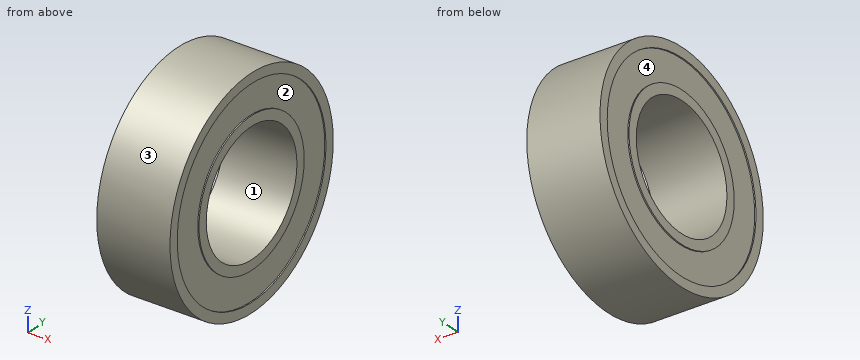
Autodesk Inventor part; units mm, degrees
ref_plane "YZ Plane" through (0, 0, 0) normal (1, 0, 0) x (0, 1, 0)
ref_plane "XZ Plane" through (0, 0, 0) normal (0, 1, 0) x (-1, 0, 0)
ref_plane "XY Plane" through (0, 0, 0) normal (0, 0, 1) x (1, 0, 0)
sketch "Эскиз1" plane through (0, 0, 0) normal (1, 0, 0) x (0, 1, 0)
  circle A0 centre (0, 0) radius 2.5
  circle A1 centre (0, 0) radius 4.5
  circle A2 centre (0, 0) radius 2.9
  circle A3 centre (0, 0) radius 4.1
  dimension "d0" = 5
  dimension "d1" = 9
  dimension "d2" = 0.4
  dimension "d3" = 0.4
extrude "Выдавливание1" add sketch "Эскиз1" along normal mid plane 3
extrude "Выдавливание2" add sketch "Эскиз1" along normal mid plane 2.9 contours A3
properties part number "roller_5_9_3"
Geometry check sheet. Reference: the model listing, model coordinates, mm. Face numbers are marked on the shaded views. A direction names the side the tool comes from. Round coordinates to 2 decimals unless told otherwise and drop trailing zeros. Order: outer loops, then holes, each group sorted by start corner. A loop starts at its lowest first (then second) coordinate and runs counter-clockwise, first axis right, second up. Notation, with made-up numbers: M 13,-7.75 L 53,-7.75 A27 cw 53,16.25 Z; hole C 72,76.5 d11. An arc over 180 degrees is marked long. Answer in a Markdown table with one row per item. Add a question column.
Item 1: Sectioned sample at C-C, the plane x = 0.75. Enter the section's corners in (y, z), plus the area to 3 significant figures.
Item 2: Set-up check for the marked faces 1 and 2: record each of +Z, -Z, +X, -X, +Y, -Y from which the full face is reachable in a straight line by a thin tool's end or side.
Item 3: Sectioned sample at D-D, the plane z = 3.75. Enter the section's corners in (x, y), plus the area to 3 significant figures.
Item 4: Sectioned sample at A-A, the plane y = 0. Enter the section's corners in (x, z), plus the area to 3 significant figures.
Item 5: Material ranges on L1, parallel to X at y = 2.25, z = 3; L2, parallel to Z at x = 1.3, y = -1.5; L3, parallel to Y at x = 0.1, z = -0.5, recorded low to high. Write a range as [from, to].
Item 6: Depth check by flat-ended pin: pin 1 Ø1.5 at (y, z) = (1, -0.5) entering from -X; pin 2 Ø1 at (x, y) = (0, 2) entering from +Z. Enter the tip coordinate at first touch or a pass-through.
Item 7: Draft check along Z on the marked faces 3 and 4. Enter one of: released by +Z, released by -Z, zero draft, split by the parting line, or undercut.
Item 8: Sectioned sample at B-B, the plane z = -0.5. Enter the section's corners in (x, y).
Filled in:
| question | item | result |
|---|---|---|
| 1 | outline | C 0,0 d9; hole C 0,0 d5 |
| 1 | area | 44.0 mm² |
| 2 | face 1 | +X, -X |
| 2 | face 2 | +X |
| 3 | outline | M -1.5,-2.49 L 1.5,-2.49 L 1.5,-1.66 L 1.45,-1.66 L 1.45,1.66 L 1.5,1.66 L 1.5,2.49 L -1.5,2.49 L -1.5,1.66 L -1.45,1.66 L -1.45,-1.66 L -1.5,-1.66 Z |
| 3 | area | 14.6 mm² |
| 4 | outline | M -1.5,-4.5 L 1.5,-4.5 L 1.5,-4.1 L 1.45,-4.1 L 1.45,-2.9 L 1.5,-2.9 L 1.5,-2.5 L -1.5,-2.5 L -1.5,-2.9 L -1.45,-2.9 L -1.45,-4.1 L -1.5,-4.1 Z; M -1.5,2.5 L 1.5,2.5 L 1.5,2.9 L 1.45,2.9 L 1.45,4.1 L 1.5,4.1 L 1.5,4.5 L -1.5,4.5 L -1.5,4.1 L -1.45,4.1 L -1.45,2.9 L -1.5,2.9 Z |
| 4 | area | 11.8 mm² |
| 5 | L1 | x = [-1.45, 1.45] |
| 5 | L2 | z = [-4.24, -2], [2, 4.24] |
| 5 | L3 | y = [-4.47, -2.45], [2.45, 4.47] |
| 6 | pin 1 | passes through |
| 6 | pin 2 | stops at z = 4.24 |
| 7 | face 3 | split by the parting line |
| 7 | face 4 | undercut |
| 8 | outline | M -1.5,-4.47 L 1.5,-4.47 L 1.5,-4.07 L 1.45,-4.07 L 1.45,-2.86 L 1.5,-2.86 L 1.5,-2.45 L -1.5,-2.45 L -1.5,-2.86 L -1.45,-2.86 L -1.45,-4.07 L -1.5,-4.07 Z; M -1.5,2.45 L 1.5,2.45 L 1.5,2.86 L 1.45,2.86 L 1.45,4.07 L 1.5,4.07 L 1.5,4.47 L -1.5,4.47 L -1.5,4.07 L -1.45,4.07 L -1.45,2.86 L -1.5,2.86 Z |
